Verification items for the finished model (mm, model axes). Face numbers are marked on the shaded views. A direction names the side the tool comes from. Round coordinates to 2 decimals unless told otherwise and drop trailing zeros. Write each loop counter-clockwise with the first axis right and the second up, starting at its lowest first coordinate (ties: lowest second). Pieces come first, ordered by that corner, then holes. Notation, with made-up numbers: M 20.5,74.25 L 42.5,74.25 A23 ccw 42.5,108.25 Z; hole C 80,5 d6. An arc over 180 degrees is marked long. One line per question, with ' | ' between items. Start each with the question number.
Q1. Cross-section at C-C (z = -27.5). Record the boundary of the cut face in (x, y), then the cut area to 3 significant figures.
Q2. Cross-section at D-D (x = 24.83). Record the boundary of the cut face in (y, z) (3 decimals), then the cut area to 3 significant figures.
Q3. Release check for a two-part mould opening along Z. For the marked faces 4, 5 and 6 record: released by +Z, released by -Z, zero draft, split by the parting line, or undercut.
Q4. Gauge pin test, flat ends, axial feed: pin 1 (8.5 mm diameter, centred on x = 52.5, y = 19.5, fed in from +Z); pin 2 (12 mm diameter, centred on x = 17.5, y = 11, fed in from -Z); pin 3 (4 mm diameter, centred on x = 30, z = -34, fed in from +Y). Record the tip position at first contact, or that the pin passes through.
Q5. Cross-section at B-B (x = 5). Record the boundary of the cut face in (y, z) (3 decimals).
Q6. Thickness scan on line 1 along Z through (x, y) = (5, 11.5) (3 decimals); line 2 along Z through (x, y) = (24.83, 5.25) (3 decimals); line 3 along Z through (x, y) = (36.61, 10) (3 decimals). Record the ranges inside material, lowest first. Write a range as from..to.
Q7. Cross-section at A-A (z = -50.5). Record the boundary of the cut face in (x, y) (3 decimals).
Q8. Tool access check on the marked faces 1, 2 and 3. Record the directions out of +Z, -Z, +X, -X, +Y, -Y that give a thin tool (end or side, any length) a straight path to the whole face; none if there is none.
from build123d import *

# Parameters (mm, degrees)
SKETCH1_R           = 2
BOSS_EXTRUDE1_DEPTH = 25
SKETCH2_W           = 55
SKETCH2_H           = 26
CUT_EXTRUDE1_DEPTH  = 10.5
FILLET1_R           = 1.55
SKETCH3_W           = 67
SKETCH3_H           = 38
SKETCH3_W_2         = 62
SKETCH3_H_2         = 33
CUT_EXTRUDE2_DEPTH  = 0.25
FILLET2_R           = 1.55
SKETCH5_R           = 2.025
CUT_EXTRUDE4_DEPTH  = 26
SKETCH6_R           = 3
CUT_EXTRUDE5_DEPTH  = 15.5
CUT_EXTRUDE6_DEPTH  = 10


with BuildPart() as part:
    # Sketch1 → Boss-Extrude1 (new body)
    with BuildSketch(Plane(origin=(0, 0, 0), x_dir=(1, 0, 0), z_dir=(0, 1, 0))):
        with BuildLine():
            Line((80, 55), (85, 55))
            Line((85, 55), (85, 0))
            Line((85, 0), (0, 0))
            Line((0, 0), (0, 55))
            Line((0, 55), (60, 55))
            ThreePointArc((60, 55), (70, 65), (80, 55))
        make_face()
        with Locations((70, 60)):
            Circle(SKETCH1_R, mode=Mode.SUBTRACT)
    extrude(amount=BOSS_EXTRUDE1_DEPTH)

    # Sketch2 → Cut-Extrude1 (cut)
    with BuildSketch(Plane(origin=(0, 25, 0), x_dir=(1, 0, 0), z_dir=(0, 1, 0))):
        with Locations((42.5, 27.5)):
            Rectangle(SKETCH2_W, SKETCH2_H)
    extrude(amount=-CUT_EXTRUDE1_DEPTH, mode=Mode.SUBTRACT)

    # Fillet1
    fillet1_edges = [part.edges().sort_by_distance(p)[0] for p in [
        (0, 12.5, -55),
        (60, 12.5, -55),
        (80, 12.5, -55),
        (85, 12.5, -55),
        (85, 12.5, 0),
        (0, 12.5, 0),
        (15, 19.75, -14.5),
        (15, 19.75, -40.5),
        (70, 19.75, -40.5),
        (70, 19.75, -14.5),
    ]]
    fillet(fillet1_edges, radius=FILLET1_R)

    # Sketch3 → Cut-Extrude2 (cut)
    with BuildSketch(Plane(origin=(0, 25, 0), x_dir=(1, 0, 0), z_dir=(0, 1, 0))):
        with Locations((42.5, 27.5)):
            Rectangle(SKETCH3_W, SKETCH3_H)
        with Locations((42.5, 27.5)):
            Rectangle(SKETCH3_W_2, SKETCH3_H_2, mode=Mode.SUBTRACT)
    extrude(amount=-CUT_EXTRUDE2_DEPTH, mode=Mode.SUBTRACT)

    # Fillet2
    fillet2_edges = [part.edges().sort_by_distance(p)[0] for p in [
        (9, 24.875, -8.5),
        (9, 24.875, -46.5),
        (76, 24.875, -46.5),
        (76, 24.875, -8.5),
        (11.5, 24.875, -44),
        (73.5, 24.875, -44),
        (73.5, 24.875, -11),
        (11.5, 24.875, -11),
    ]]
    fillet(fillet2_edges, radius=FILLET2_R)

    # Sketch5 → Cut-Extrude4 (cut, through all)
    with BuildSketch(Plane(origin=(0, 25, 0), x_dir=(1, 0, 0), z_dir=(0, 1, 0))):
        with Locations((5, 42.45)):
            Circle(SKETCH5_R)
        with Locations((5, 12.55)):
            Circle(SKETCH5_R)
        with Locations((13.05, 4.5)):
            Circle(SKETCH5_R)
        with Locations((71.95, 4.5)):
            Circle(SKETCH5_R)
        with Locations((24.83, 4.5)):
            Circle(SKETCH5_R)
        with Locations((36.61, 4.5)):
            Circle(SKETCH5_R)
        with Locations((48.39, 4.5)):
            Circle(SKETCH5_R)
        with Locations((60.17, 4.5)):
            Circle(SKETCH5_R)
        with Locations((5, 32.483333333)):
            Circle(SKETCH5_R)
        with Locations((5, 22.516666667)):
            Circle(SKETCH5_R)
        with Locations((80, 42.45)):
            Circle(SKETCH5_R)
        with Locations((80, 12.55)):
            Circle(SKETCH5_R)
        with Locations((80, 22.516666667)):
            Circle(SKETCH5_R)
        with Locations((80, 32.483333333)):
            Circle(SKETCH5_R)
        with Locations((13.05, 50.5)):
            Circle(SKETCH5_R)
        with Locations((24.83, 50.5)):
            Circle(SKETCH5_R)
        with Locations((36.61, 50.5)):
            Circle(SKETCH5_R)
        with Locations((48.39, 50.5)):
            Circle(SKETCH5_R)
        with Locations((60.17, 50.5)):
            Circle(SKETCH5_R)
        with Locations((71.95, 50.5)):
            Circle(SKETCH5_R)
    extrude(amount=-CUT_EXTRUDE4_DEPTH, mode=Mode.SUBTRACT)

    # Sketch6 → Cut-Extrude5 (cut, through all)
    with BuildSketch(Plane(origin=(0, 14.5, 0), x_dir=(1, 0, 0), z_dir=(0, 1, 0))):
        with Locations((24.83, 27.5)):
            Circle(SKETCH6_R)
    extrude(amount=-CUT_EXTRUDE5_DEPTH, mode=Mode.SUBTRACT)

    # Sketch7 → Cut-Extrude6 (cut)
    with BuildSketch(Plane(origin=(0, 25, 0), x_dir=(1, 0, 0), z_dir=(0, 1, 0))):
        with BuildLine():
            Line((58.554476858, 55), (81.445523142, 55))
            ThreePointArc((81.445523142, 55), (80.425698015, 55.382756791), (79.909543846, 56.341991342))
            ThreePointArc((79.909543846, 56.341991342), (70, 65), (60.090456154, 56.341991342))
            ThreePointArc((60.090456154, 56.341991342), (59.574301985, 55.382756791), (58.554476858, 55))
        make_face()
    extrude(amount=-CUT_EXTRUDE6_DEPTH, mode=Mode.SUBTRACT)


solid = part.part
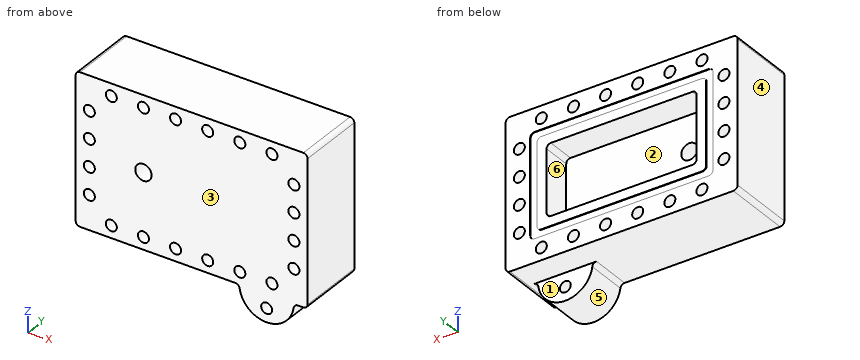
Determined:
1) outline: M 0,0 L 21.83,0 L 21.83,14.5 L 15,14.5 L 15,25 L 11.5,25 L 11.5,24.75 L 9,24.75 L 9,25 L 0,25 Z; M 27.83,0 L 85,0 L 85,25 L 76,25 L 76,24.75 L 73.5,24.75 L 73.5,25 L 70,25 L 70,14.5 L 27.83,14.5 Z | area: 1,460 mm²
2) outline: M 0,-55 L 25,-55 L 25,-52.525 L 0,-52.525 Z; M 0,-48.475 L 25,-48.475 L 25,-46.5 L 24.75,-46.5 L 24.75,-44 L 25,-44 L 25,-40.5 L 14.5,-40.5 L 14.5,-30.5 L 0,-30.5 Z; M 0,-24.5 L 14.5,-24.5 L 14.5,-14.5 L 25,-14.5 L 25,-11 L 24.75,-11 L 24.75,-8.5 L 25,-8.5 L 25,-6.525 L 0,-6.525 Z; M 0,-2.475 L 25,-2.475 L 25,0 L 0,0 Z | area: 811 mm²
3) face 4: zero draft | face 5: released by -Z | face 6: undercut
4) pin 1: stops at z = 0 | pin 2: stops at z = -55 | pin 3: stops at y = 14.5
5) outline: M 0,-55 L 25,-55 L 25,-44.475 L 0,-44.475 Z; M 0,-40.425 L 25,-40.425 L 25,-34.508 L 0,-34.508 Z; M 0,-30.458 L 25,-30.458 L 25,-24.542 L 0,-24.542 Z; M 0,-20.492 L 25,-20.492 L 25,-14.575 L 0,-14.575 Z; M 0,-10.525 L 25,-10.525 L 25,0 L 0,0 Z
6) line 1: z = -55..-44.475, -40.425..-34.508, -30.458..-24.542, -20.492..-14.575, -10.525..0 | line 2: z = -55..-52.525, -48.475..-30.5, -24.5..-6.525, -2.475..0 | line 3: z = -55..-52.525, -48.475..-6.525, -2.475..0
7) outline: M 0,0 L 11.025,0 L 11.025,25 L 0,25 Z; M 15.075,0 L 22.805,0 L 22.805,25 L 15.075,25 Z; M 26.855,0 L 34.585,0 L 34.585,25 L 26.855,25 Z; M 38.635,0 L 46.365,0 L 46.365,25 L 38.635,25 Z; M 50.415,0 L 58.145,0 L 58.145,25 L 50.415,25 Z; M 62.195,0 L 69.925,0 L 69.925,25 L 62.195,25 Z; M 73.975,0 L 85,0 L 85,25 L 73.975,25 Z
8) face 1: -Z, +X, -X, +Y | face 2: +Y | face 3: +Z, -Z, +X, -X, -Y
